Could you check a few things on this model? Use its own coordinates, in mm. A direction names the side the tool comes from. Give positions to 0.01 mm unless a question says otherwise; leave off trailing zeros. Order: outer loops, then holes, each group sorted by start corner. A loop starts at its lowest first (then second) coordinate and runs counter-clockwise, first axis right, second up.
from build123d import *

# Parameters (mm, degrees)
SKETCH1_W                = 25
SKETCH1_H                = 6.75
BOSS_EXTRUDE1_DEPTH      = 6.5
BOSS_EXTRUDE4_DEPTH      = 6.5
BOSS_EXTRUDE3_DEPTH      = 6
BOSS_EXTRUDE3_DEPTH_BACK = 4.95
SKETCH4_W                = 2.3
SKETCH4_H                = 4.5
CUT_EXTRUDE1_DEPTH       = 23
SKETCH6_R                = 2.55
CUT_EXTRUDE2_DEPTH       = 10
BOSS_EXTRUDE5_DEPTH      = 1.575
CUT_EXTRUDE3_DEPTH       = 3
SKETCH9_R                = 0.8
CUT_EXTRUDE4_DEPTH       = 10.95
BOSS_EXTRUDE6_DEPTH      = 0.25


with BuildPart() as part:
    # Sketch1 → Boss-Extrude1 (new body)
    with BuildSketch(Plane(origin=(0, 0, 0), x_dir=(1, 0, 0), z_dir=(0, 1, 0))):
        with Locations((12.5, -3.375)):
            Rectangle(SKETCH1_W, SKETCH1_H)
    extrude(amount=BOSS_EXTRUDE1_DEPTH)

    # Sketch5 → Boss-Extrude4 (add)
    with BuildSketch(Plane(origin=(0, 6.5, 0), x_dir=(1, 0, 0), z_dir=(0, 1, 0))):
        Polygon((-5.715767665, -3.375), (-2.857883832, -8.325), (2.857883832, -8.325), (5.715767665, -3.375), (2.857883832, 1.575), (-2.857883832, 1.575), align=None)
    extrude(amount=-BOSS_EXTRUDE4_DEPTH)

    # Sketch3 → Boss-Extrude3 (add, two sides)
    with BuildSketch(Plane.XY.offset(3.375)) as boss_extrude3_sk:
        Polygon((19.993989967, 13.671468913), (24.823619098, 14.965564139), (30, -4.352952387), (25.170370869, -5.647047613), align=None)
    extrude(amount=BOSS_EXTRUDE3_DEPTH)
    extrude(boss_extrude3_sk.sketch, amount=-BOSS_EXTRUDE3_DEPTH_BACK)

    # Sketch4 → Cut-Extrude1 (cut)
    with BuildSketch(Plane(origin=(-2.078523862, 7.757156658, 0), x_dir=(0.965925826, 0.258819045, 0), z_dir=(-0.258819045, 0.965925826, 0))):
        with Locations((26.701147808, -2.675)):
            Rectangle(SKETCH4_W, SKETCH4_H)
    extrude(amount=-CUT_EXTRUDE1_DEPTH, mode=Mode.SUBTRACT)

    # Sketch6 → Cut-Extrude2 (cut)
    with BuildSketch(Plane(origin=(0, 6.5, 0), x_dir=(1, 0, 0), z_dir=(0, 1, 0))):
        with Locations((0, -3.335615973)):
            Circle(SKETCH6_R)
    extrude(amount=-CUT_EXTRUDE2_DEPTH, mode=Mode.SUBTRACT)

    # Sketch7 → Boss-Extrude5 (add)
    with BuildSketch(Plane(origin=(0, 0, -1.575), x_dir=(-1, 0, 0), z_dir=(0, 0, -1))):
        Polygon((-2.857883832, 0), (-23.657249021, 0), (-25.170370869, -5.647047613), (-30, -4.352952387), (-24.823619098, 14.965564139), (-19.993989967, 13.671468913), (-21.91557927, 6.5), (-2.857883832, 6.5), align=None)
    extrude(amount=-BOSS_EXTRUDE5_DEPTH)

    # Sketch8 → Cut-Extrude3 (cut)
    with BuildSketch(Plane(origin=(0, 0, 0), x_dir=(-1, 0, 0), z_dir=(0, -1, 0))):
        Polygon((-4.67653718, -11.475), (4.67653718, -11.475), (9.353074361, -3.375), (4.67653718, 4.725), (-4.67653718, 4.725), (-9.353074361, -3.375), align=None)
    extrude(amount=-CUT_EXTRUDE3_DEPTH, mode=Mode.SUBTRACT)

    # Sketch9 → Cut-Extrude4 (cut)
    with BuildSketch(Plane(origin=(0, 0, -1.575), x_dir=(-1, 0, 0), z_dir=(0, 0, -1))):
        with Locations((-28.356067858, -3.240528406)):
            Circle(SKETCH9_R)
        with Locations((-27.061972633, 1.589100725)):
            Circle(SKETCH9_R)
        with Locations((-25.767877407, 6.418729856)):
            Circle(SKETCH9_R)
        with Locations((-24.473782182, 11.248358988)):
            Circle(SKETCH9_R)
    extrude(amount=-CUT_EXTRUDE4_DEPTH, mode=Mode.SUBTRACT)

    # Sketch10 → Boss-Extrude6 (add)
    with BuildSketch(Plane.XY.offset(6.75)):
        Polygon((11.821517388, 5.121255448), (12.792571074, 5.121255448), (12.792571074, 1.621255448), (12.164365946, 1.621255448), (12.164365946, 4.537922115), (11.446417228, 4.537922115), align=None)
        with BuildLine():
            Line((14.519434055, 5.121255448), (16.113083895, 5.121255448))
            Line((16.113083895, 5.121255448), (16.113083895, 4.537922115))
            Line((16.113083895, 4.537922115), (15.017230529, 4.537922115))
            Line((15.017230529, 4.537922115), (14.880511779, 3.876063141))
            add(Edge.make_bspline(
                [(14.880511779, 3.876063141), (14.899141666, 3.881251799), (14.93588363, 3.8914849), (14.991235445, 3.901747406), (15.044879068, 3.908399236), (15.080079686, 3.909286501), (15.097158414, 3.909716987)],
                knots=[0, 0, 0, 0, 5.799e-05, 0.000114368, 0.000168722, 0.000219947, 0.000219947, 0.000219947, 0.000219947], degree=3))
            add(Edge.make_bspline(
                [(15.097158414, 3.909716987), (15.134374752, 3.908864196), (15.207736352, 3.907183157), (15.315055064, 3.891224618), (15.41781907, 3.866090403), (15.515713902, 3.830243826), (15.608643929, 3.78358858), (15.696721801, 3.727148811), (15.780055618, 3.66082539), (15.857165021, 3.584576793), (15.928016362, 3.500854107), (15.989617562, 3.410299164), (16.042228831, 3.314203188), (16.084074015, 3.211968849), (16.117101802, 3.104238248), (16.140968418, 2.990942348), (16.15508194, 2.871946875), (16.156985062, 2.790764772), (16.157955689, 2.749360416)],
                knots=[0, 0, 0, 0, 0.000111586, 0.000219961, 0.00032471, 0.000428519, 0.000531991, 0.000636043, 0.000741817, 0.000850891, 0.00096086, 0.001070345, 0.001178899, 0.001288921, 0.00140114, 0.00151651, 0.001635827, 0.001760022, 0.001760022, 0.001760022, 0.001760022], degree=3))
            add(Edge.make_bspline(
                [(16.157955689, 2.749360416), (16.156769568, 2.707486025), (16.154429003, 2.62485561), (16.139158961, 2.503359672), (16.112207063, 2.386993992), (16.075185934, 2.275447061), (16.026412967, 2.169538723), (15.967756798, 2.068171845), (15.898225712, 1.972098843), (15.818502044, 1.882304581), (15.73183196, 1.800230902), (15.639548779, 1.728030529), (15.54230082, 1.6672745), (15.440085734, 1.618173357), (15.333489963, 1.579325407), (15.222481155, 1.551045953), (15.106519819, 1.534829258), (15.027797139, 1.53262981), (14.987783414, 1.531511859)],
                knots=[0, 0, 0, 0, 0.000125626, 0.000247897, 0.00036661, 0.000483454, 0.000599853, 0.000715778, 0.000834286, 0.000954987, 0.001075509, 0.001191914, 0.001305919, 0.001418808, 0.001531482, 0.001645754, 0.001761863, 0.001881886, 0.001881886, 0.001881886, 0.001881886], degree=3))
            add(Edge.make_bspline(
                [(14.987783414, 1.531511859), (14.95200033, 1.532426412), (14.881428601, 1.534230104), (14.777479542, 1.545316541), (14.677261106, 1.564917466), (14.581305344, 1.593285081), (14.488602639, 1.628199138), (14.400224662, 1.671865764), (14.315685761, 1.723453489), (14.235225994, 1.782020834), (14.160152719, 1.847994677), (14.091633788, 1.920214415), (14.029254379, 1.997769753), (13.974349314, 2.08161749), (13.927090704, 2.171633744), (13.885180804, 2.266757653), (13.850877131, 2.367982614), (13.833469005, 2.438157381), (13.824622356, 2.473819551)],
                knots=[0, 0, 0, 0, 0.000107354, 0.000211725, 0.000313201, 0.000413265, 0.000511575, 0.000610032, 0.000708511, 0.000808359, 0.000908217, 0.001007897, 0.001106663, 0.001206422, 0.001308044, 0.00141134, 0.001517986, 0.001628185, 0.001628185, 0.001628185, 0.001628185], degree=3))
            Line((13.824622356, 2.473819551), (14.542571074, 2.473819551))
            add(Edge.make_bspline(
                [(14.542571074, 2.473819551), (14.555695194, 2.44910712), (14.581200423, 2.401081329), (14.629717008, 2.337319877), (14.684028245, 2.282946849), (14.743644216, 2.23743101), (14.808951196, 2.203331319), (14.87728805, 2.17747169), (14.949513264, 2.162528368), (14.998701823, 2.160660305), (15.023540625, 2.159716987)],
                knots=[0, 0, 0, 0, 8.3833e-05, 0.00016292, 0.000239268, 0.000313868, 0.00038695, 0.000459491, 0.000532506, 0.000606986, 0.000606986, 0.000606986, 0.000606986], degree=3))
            add(Edge.make_bspline(
                [(15.023540625, 2.159716987), (15.040852937, 2.160368356), (15.074915202, 2.161649936), (15.125100563, 2.168429817), (15.173004696, 2.181270757), (15.218983754, 2.199052474), (15.263161251, 2.221228283), (15.304903887, 2.249223798), (15.344937907, 2.281447673), (15.382653832, 2.318424679), (15.416813589, 2.35964544), (15.44676796, 2.403939957), (15.473551298, 2.450323998), (15.493390125, 2.500634949), (15.509636448, 2.553370509), (15.521600897, 2.608928478), (15.528751005, 2.667373743), (15.529412913, 2.707272687), (15.529750561, 2.727625641)],
                knots=[0, 0, 0, 0, 5.1959e-05, 0.00010223, 0.000151548, 0.000200376, 0.000249918, 0.000299504, 0.000350859, 0.000403908, 0.00045768, 0.000511159, 0.000564208, 0.00061798, 0.000672982, 0.000729638, 0.000788252, 0.000849286, 0.000849286, 0.000849286, 0.000849286], degree=3))
            add(Edge.make_bspline(
                [(15.529750561, 2.727625641), (15.529358682, 2.747506156), (15.528595879, 2.786204063), (15.52228582, 2.843026451), (15.510997246, 2.896940614), (15.495616468, 2.948359494), (15.475927235, 2.996970851), (15.451865677, 3.043064042), (15.423328999, 3.086406084), (15.390163995, 3.126114575), (15.354797176, 3.162536333), (15.316801847, 3.194390511), (15.276520328, 3.220827268), (15.235204316, 3.243907326), (15.191204624, 3.260704489), (15.14551063, 3.272272075), (15.098170386, 3.280759905), (15.065880633, 3.281258596), (15.049482132, 3.281511859)],
                knots=[0, 0, 0, 0, 5.9632e-05, 0.000116076, 0.000171216, 0.000224671, 0.00027688, 0.000328311, 0.000380426, 0.000432223, 0.00048329, 0.000532573, 0.000580604, 0.000627663, 0.000674276, 0.000721381, 0.000768985, 0.000818109, 0.000818109, 0.000818109, 0.000818109], degree=3))
            add(Edge.make_bspline(
                [(15.049482132, 3.281511859), (15.031669548, 3.28083597), (14.995969309, 3.279481344), (14.942927689, 3.268459116), (14.890525603, 3.250621017), (14.838471643, 3.226010532), (14.787282533, 3.193803172), (14.735607368, 3.156027632), (14.685175827, 3.10993916), (14.65311005, 3.075612361), (14.636521395, 3.057854006)],
                knots=[0, 0, 0, 0, 5.34e-05, 0.000107026, 0.00016179, 0.000219183, 0.000279308, 0.000342972, 0.00041098, 0.000483874, 0.000483874, 0.000483874, 0.000483874], degree=3))
            Line((14.636521395, 3.057854006), (14.107875561, 3.179148077))
            Line((14.107875561, 3.179148077), (14.519434055, 5.121255448))
        make_face()
        Polygon((17.234878766, 5.210999038), (17.8182121, 5.210999038), (17.672378766, 4.537922115), (18.215748157, 5.013983814), (18.491289023, 4.537922115), (17.773340305, 4.335999038), (18.491289023, 4.134075961), (18.180692068, 3.647497435), (17.6541496, 4.134075961), (17.8182121, 3.460999038), (17.234878766, 3.460999038), (17.412262581, 4.134075961), (16.873801042, 3.647497435), (16.561801843, 4.134075961), (17.279750561, 4.335999038), (16.561801843, 4.537922115), (16.873801042, 5.036419711), (17.412262581, 4.537922115), align=None)
    extrude(amount=BOSS_EXTRUDE6_DEPTH)


solid = part.part
Item 1: Imagine slicing it at A-A on x = 0. List the corners of the cut face in (y, z) for me (3 decimals), then the cut area to 3 significant figures.
Findings:
outline: (3, -1.575) - (6.5, -1.575) - (6.5, 0.786) - (3, 0.786) - close; (3, 5.886) - (6.5, 5.886) - (6.5, 8.325) - (3, 8.325) - close
area: 16.8 mm2
Item 2: We'd pull the mould along Y, two halves only. Please class faces 4 (the flat face through (15, 0, 3)), 5 (the flat face through (26, 5, 4.925)), 6 (the cylindrical face through (27.86, 1.62, -0.59)), 7 (the cylindrical face through (28.946, -2.7, 7.119)): +Y half, -Y half, draft (parallel to the pull), parting line (faces both ways), or undercut.
Findings:
face 4: -Y half
face 5: draft
face 6: undercut
face 7: undercut
Item 3: Please list where these lines run through material, in increasing order: line 1 along Z through (x, y) = (0, 4.6) (3 decimals); line 2 along Y through (x, z) = (2, 1.25); line 3 along X through (y, z) = (3.25, 2.75).
Findings:
line 1: z = -1.575 to 0.786, 5.886 to 8.325
line 2: y = 3 to 6.5
line 3: x = -5.35 to -2.48, 2.48 to 25.58
Item 4: Imagine slicing it at D-D on y = -0.5. List the corners of the cut face in (x, z) for me (3 decimals).
Findings:
outline: (23.791, -1.575) - (28.968, -1.575) - (28.968, 0.425) - (26.586, 0.425) - (26.586, 4.925) - (28.968, 4.925) - (28.968, 9.375) - (23.791, 9.375) - close
Item 5: Imagine slicing it at B-B on z = 2. List the corners of the cut face in (x, y) for me, then the cut area to 3 significant figures.
Findings:
outline: (-4.92, 3) - (-2.17, 3) - (-2.17, 6.5) - (-4.92, 6.5) - close; (2.17, 3) - (8.56, 3) - (8.56, 0) - (23.66, 0) - (25.17, -5.65) - (27.78, -4.95) - (22.6, 14.37) - (19.99, 13.67) - (21.92, 6.5) - (2.17, 6.5) - close
area: 178 mm2
Item 6: For pin 1 (4.5 mm diameter, centred on x = 0, z = 3.34, fed in from -Y) (3 decimals); pin 2 (12 mm diameter, centred on x = 7, y = 6, fed in from +Z) (3 decimals); pin 3 (3 mm diameter, centred on x = 9.5, z = 2, fed in from +Y); pin 4 (1.5 mm diameter, centred on y = -1.5, z = 1, fed in from +X), each with a flat end and sliding along its axis, tell me the tip position at first contact or that it passes through.
Findings:
pin 1: passes through
pin 2: stops at z = 8.325
pin 3: stops at y = 6.5
pin 4: stops at x = 29.36
Item 7: For faces 1 (the flat face through (25.154, 4.846, 2.706)), 2 (the flat face through (15.3, 3.4, 7)), 3 (the flat face through (8, 6.5, 3)), which set-ups out of +Z, -Z, +X, -X, +Y, -Y let a thin tool reach every point of the face, with its end or its side?
Findings:
face 1: +X, +Y
face 2: +Z, +Y, -Y
face 3: +Z, -Z, -X
Item 8: Imagine slicing it at C-C on x = 5. List the corners of the cut face in (y, z) for me (3 decimals).
Findings:
outline: (3, -1.575) - (6.5, -1.575) - (6.5, 6.75) - (3, 6.75) - close
